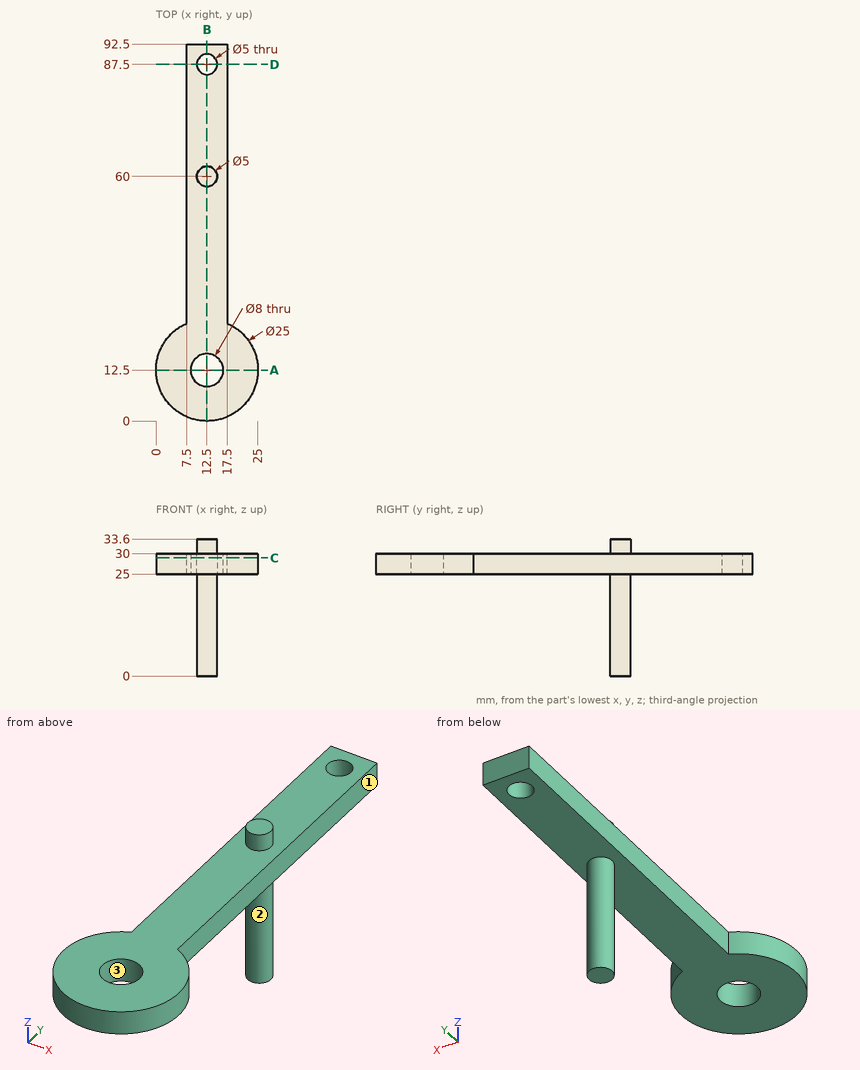
Print and shaded views of the part. All mm, measured from the part's lowest x, y and z. A direction names the side the tool comes from. Round coordinates to 2 decimals unless told otherwise and drop trailing zeros. Write each loop counter-clockwise with the first axis right and the second up, starting at its lowest first coordinate (ties: lowest second). Pieces come first, ordered by that corner, then holes. Notation, with made-up numbers: (18, 85.25) - (46, 85.25) arc R33 cw to (46, 123.25) - close; hole circle Ø8 at (76.25, 53). An arc over 180 degrees is marked (long way). Write each question's results on one line, items separated by ' | '. Start each with the question number.
Item 1: Wall check: L1, parallel to Y at x = 12.5, z = 26.8; L2, parallel to X at y = 30, z = 26; L3, parallel to Z at x = 9.5, y = 41. Give the ranges that are in metal, low to high. Write a range as [from, to].
Item 2: Saw through at A-A (y = 12.5). Write the cut outline in (x, z).
Item 3: Saw through at D-D (y = 87.5). Write the cut outline in (x, z), and give its area (3 significant figures).
Item 4: Drop flat-ended pins along their axis: P1, Ø5, axis at y = 24, z = 28.5, coming from the -X side; P2, Ø8, axis at x = 12.5, y = 87.5, coming from the +Z side; P3, Ø10, axis at x = 13.5, z = 5, coming from the +Y side. Give the stop position or say it passes through.
Item 5: Saw through at B-B (x = 12.5). Write the cut outline in (y, z), and give its area (4 significant figures).
Item 6: Which spindle directions (+Z, -Z, +X, -X, +Y, -Y) get a long thin tool onto all of the face, cutting with end or side? Do the marked faces 1, 2 and 3. Say none if no direction does.
Item 7: Saw through at C-C (z = 29). Write the cut outline in (x, y).
Results are:
1) L1: y = [0, 8.5], [16.5, 85], [90, 92.5] | L2: x = [7.5, 17.5] | L3: z = [25, 30]
2) outline: (0, 25) - (8.5, 25) - (8.5, 30) - (0, 30) - close; (16.5, 25) - (25, 25) - (25, 30) - (16.5, 30) - close
3) outline: (7.5, 25) - (10, 25) - (10, 30) - (7.5, 30) - close; (15, 25) - (17.5, 25) - (17.5, 30) - (15, 30) - close | area: 25.0 mm²
4) P1: stops at x = 3.83 | P2: stops at z = 30 | P3: stops at y = 62.5
5) outline: (0, 25) - (8.5, 25) - (8.5, 30) - (0, 30) - close; (16.5, 25) - (57.5, 25) - (57.5, 0) - (62.5, 0) - (62.5, 25) - (85, 25) - (85, 30) - (62.5, 30) - (62.5, 33.6) - (57.5, 33.6) - (57.5, 30) - (16.5, 30) - close; (90, 25) - (92.5, 25) - (92.5, 30) - (90, 30) - close | area: 540.5 mm²
6) face 1: +Z, -Z, +X, +Y | face 2: -Z | face 3: +Z, -Z
7) outline: (7.5, 23.96) arc R12.5 ccw (long way) to (17.5, 23.96) - (17.5, 92.5) - (7.5, 92.5) - close; hole circle Ø8 at (12.5, 12.5); hole circle Ø5 at (12.5, 87.5)
